from build123d import *

# Parameters (mm, degrees)
BOSS_EXTRU_1_DEPTH           = 15
ENL_V_MAT_EXTRU_1_DEPTH      = 3
ENL_V_MAT_EXTRU_1_DEPTH_BACK = 2.8
D_GAGEMENT_M42_D             = 4.8
ENL_V_MAT_EXTRU_2_REACH      = 46.643
ESQUISSE11_W                 = 17.14444817
ESQUISSE11_H                 = 8.906875476
ESQUISSE11_R                 = 2.1
BOSS_EXTRU_2_DEPTH           = 3


# Read off the part's stored shape, not the designer's step: Boss.-Extru.1
with BuildPart() as part:
    # Boss.-Extru.1 outline → Boss.-Extru.1 (new body)
    with BuildSketch(Plane.XY):
        with BuildLine():
            Line((5.987288652, 22.39857253), (-11.866871143, 15.900189807))
            Line((-11.866871143, 15.900189807), (-10.941224384, 13.356996238))
            ThreePointArc((-10.941224384, 13.356996238), (-10.69253266, 10.921872002), (-11.629511209, 8.660512054))
            ThreePointArc((-11.629511209, 8.660512054), (-12.486015657, 7.372205437), (-13.200388341, 5.99997897))
            ThreePointArc((-13.200388341, 5.99997897), (-19.184502611, 0), (-13.200388341, -5.99997897))
            ThreePointArc((-13.200388341, -5.99997897), (-2.413103056, -14.297794713), (10.5, -10))
            Line((10.5, -10), (20.356157589, -10))
            Line((20.356157589, -10), (20.356157589, -6))
            Line((20.356157589, -6), (10.356157589, -6))
            ThreePointArc((10.356157589, -6), (9.887116013, -6.116823913), (9.527664982, -6.44))
            ThreePointArc((9.527664982, -6.44), (-1.63993081, -11.38247016), (-10.958116089, -3.488508533))
            ThreePointArc((-10.958116089, -3.488508533), (-11.458744879, -2.899966328), (-12.229372464, -2.843892826))
            ThreePointArc((-12.229372464, -2.843892826), (-16.184502611, 0), (-12.229372464, 2.843892826))
            ThreePointArc((-12.229372464, 2.843892826), (-11.458744879, 2.899966328), (-10.958116089, 3.488508533))
            ThreePointArc((-10.958116089, 3.488508533), (-1.63993081, 11.38247016), (9.527664982, 6.44))
            ThreePointArc((9.527664982, 6.44), (9.887116013, 6.116823913), (10.356157589, 6))
            Line((10.356157589, 6), (20.356157589, 6))
            Line((20.356157589, 6), (20.356157589, 10))
            Line((20.356157589, 10), (14.001037691, 10))
            ThreePointArc((14.001037691, 10), (11.133155509, 10.904239779), (9.302574587, 13.289899283))
            Line((9.302574587, 13.289899283), (5.987288652, 22.39857253))
        make_face()
    extrude(amount=BOSS_EXTRU_1_DEPTH)

    # Esquisse5 → Enlèv. mat.-Extru.1 (cut, two sides: drawn at the far end of the back side and taken through both)
    with BuildSketch(Plane(origin=(0, 10, 0), x_dir=(1, 0, 0), z_dir=(0, 1, 0)).offset(-ENL_V_MAT_EXTRU_1_DEPTH_BACK)):
        Polygon((18.356157589, -9.520725942), (18.356157589, -5.479274058), (14.856157589, -3.458548116), (11.356157589, -5.479274058), (11.356157589, -9.520725942), (14.856157589, -11.541451884), align=None)
    extrude(amount=ENL_V_MAT_EXTRU_1_DEPTH + ENL_V_MAT_EXTRU_1_DEPTH_BACK, mode=Mode.SUBTRACT)

    # Dégagement M42 (through all)
    with Locations(Plane(origin=(0, 10, 0), x_dir=(1, 0, 0), z_dir=(0, 1, 0))):
        with Locations((14.856157589, -7.5)):
            Hole(D_GAGEMENT_M42_D / 2)

    # Esquisse10 → Enlèv. mat.-Extru.2 (cut, up to next)
    with BuildSketch(Plane(origin=(-6.498382723, 17.854159795, 0), x_dir=(0.9396926207859082, 0.3420201433256695, 0), z_dir=(-0.3420201433256695, 0.9396926207859082, 0)), mode=Mode.PRIVATE) as enl_v_mat_extru_2_sk1:
        Polygon((-4.213026048, -9.520725942), (-0.713026048, -11.541451884), (2.786973952, -9.520725942), (2.786973952, -5.479274058), (-0.713026048, -3.458548116), (-4.213026048, -5.479274058), align=None)
    enl_v_mat_extru_2_tool1 = extrude(enl_v_mat_extru_2_sk1.sketch, amount=-ENL_V_MAT_EXTRU_2_REACH, mode=Mode.PRIVATE) & part.part
    # Esquisse10 → Enlèv. mat.-Extru.2 (cut, up to next)
    with BuildSketch(Plane(origin=(-6.498382723, 17.854159795, 0), x_dir=(0.9396926207859082, 0.3420201433256695, 0), z_dir=(-0.3420201433256695, 0.9396926207859082, 0)), mode=Mode.PRIVATE) as enl_v_mat_extru_2_sk2:
        Polygon((11.832491793, -9.439751676), (11.739607101, -5.399367318), (8.194089259, -3.459615641), (4.74145611, -5.560248324), (4.834340802, -9.600632682), (8.379858644, -11.540384359), align=None)
    enl_v_mat_extru_2_tool2 = extrude(enl_v_mat_extru_2_sk2.sketch, amount=-ENL_V_MAT_EXTRU_2_REACH, mode=Mode.PRIVATE) & part.part
    add(enl_v_mat_extru_2_tool1.solids().sort_by_distance((-7.168408, 17.610291, 7.5))[0], mode=Mode.SUBTRACT)
    add(enl_v_mat_extru_2_tool2.solids().sort_by_distance((1.288826, 20.688472, 7.5))[0], mode=Mode.SUBTRACT)

    # Esquisse11 → Boss.-Extru.2 (add)
    with BuildSketch(Plane(origin=(-6.498382723, 17.854159795, 0), x_dir=(0.9396926207859082, 0.3420201433256694, 0), z_dir=(-0.3420201433256694, 0.9396926207859083, 0))):
        with Locations((3.831914323, -7.577227244)):
            Rectangle(ESQUISSE11_W, ESQUISSE11_H)
        with Locations(Location((-0.713026048, -7.5, 0), (0, 0, 180))):
            Circle(ESQUISSE11_R, mode=Mode.SUBTRACT)
        with Locations(Location((8.283576678, -7.5, 0), (0, 0, 180))):
            Circle(ESQUISSE11_R, mode=Mode.SUBTRACT)
    extrude(amount=-BOSS_EXTRU_2_DEPTH)


solid = part.part
Design review of the part built by this model. Coordinates are the model's own, in mm. A direction names the side the tool comes from. Give positions to 0.01 mm unless a question says otherwise; leave off trailing zeros. Loops run counter-clockwise (first coordinate to the right, second up) from the corner with the lowest first, then second, coordinate; pieces in that order, holes last. Notation, with made-up numbers: M 86.5,16 L 90.5,16 A21 ccw 90.5,39 Z; hole C -14.5,79.5 d7. An arc over 180 degrees is marked long. Answer as a JSON object with one key per item and string values.
Item 1: Wall thickness on line 1 along Y through (x, z) = (18, 7.5); line 2 along X through (y, z) = (0, 8.25); line 3 along Y through (x, z) = (16, 3.5): over which ranges is each line inside the solid? List them lowest first.
Output values:
{"line 1": "y = -10 to -6, 6 to 7.2", "line 2": "x = -19.18 to -16.18", "line 3": "y = -10 to -6, 6 to 10"}
Item 2: We need section C-C (x = 3). Count the separate pieces of the cut face and the enclosed holes in it, and give its area (3 significant figures).
Output values:
{"separate pieces": "3", "enclosed holes": "0", "area": "138 mm2"}
Item 3: We need section B-B (z = 14). State the section outline as (x, y) points.
Output values:
{"outline": "M -13.2,-6 A14.5 ccw 10.5,-10 L 20.36,-10 L 20.36,-6 L 10.36,-6 A1 ccw 9.53,-6.44 A11.5 cw -10.96,-3.49 A1 ccw -12.23,-2.84 A3 cw long -12.23,2.84 A1 ccw -10.96,3.49 A11.5 cw 9.53,6.44 A1 ccw 10.36,6 L 20.36,6 L 20.36,10 L 14,10 A5 cw 9.3,13.29 L 5.99,22.4 L -11.87,15.9 L -10.94,13.36 A5 cw -11.63,8.66 A14.5 ccw -13.2,6 A6 ccw Z"}
Item 4: For P1, Ø2, axis at y = 17, z = 4.5, coming from the +X side; P2, Ø7, axis at x = 17, z = 5.5, coming from the +Y side; P3, Ø8, axis at x = 14.5, z = 7, coming from the +Y side, all flat-tipped, find the tip position at first contact; note any pin that passes through.
Output values:
{"P1": "stops at x = 8.32", "P2": "stops at y = 10", "P3": "stops at y = 11.43"}
Item 5: Mouldability with a two-part tool opening along X and no side actions: class faces 1 (the face through (1.774, 14.371, 10.557)), 2 (the face through (-2.608, -14.263, 7.395)), 3 (the face through (-11.41, 14.65, 7.4)), 4 (the face through (-3.66, 13.15, 4.48)) as pulls with the +X half, pulls with the -X half, needs draft (parallel to the pull), parting line crosses it, or undercut.
Output values:
{"face 1": "undercut", "face 2": "parting line crosses it", "face 3": "pulls with the -X half", "face 4": "undercut"}
Item 6: Machinability: for faces 5 (the face through (20.356, -8, 7)), 6 (the face through (19, 10, 7)), 7 (the face through (-3.704, 13.138, 10.545)), 8 (the face through (-11.469, 2.895, 7.395)), which of the approach directions +Z, -Z, +X, -X, +Y, -Y give a long, thin tool a straight path to every point of the face, cutting with its end or side? Answer none if there is none.
Output values:
{"face 5": "+Z, -Z, +X, +Y, -Y", "face 6": "+Z, -Z, +X, +Y", "face 7": "none", "face 8": "+Z, -Z"}
Item 7: We need section A-A (y = -7.5). State the section outline as (x, z) points.
Output values:
{"outline": "M -12.41,0 L -8.72,0 L -8.72,15 L -12.41,15 Z; M 8.72,0 L 20.36,0 L 20.36,15 L 8.72,15 Z; hole C 14.86,7.5 d4.8"}
Item 8: We need section D-D (y = 0). State the section outline as (x, z) points, and give its area (3 significant figures).
Output values:
{"outline": "M -19.18,0 L -16.18,0 L -16.18,15 L -19.18,15 Z", "area": "45.0 mm2"}
